Source: CAD feature listing. Evaluate the final solid. Frame: model axes, mm. A direction names the side the tool comes from. Give positions to 0.01 mm unless a question says otherwise; leave off trailing zeros. Write each loop counter-clockwise with the first axis right and the second up, starting at its lowest first coordinate (ties: lowest second). Pieces come first, ordered by that corner, then holes. Notation, with made-up numbers: (82, -3.5) - (100, -3.5) arc R21 cw to (100, 33.5) - close; hole circle Ø6 at (-31, 3). An arc over 180 degrees is marked (long way). One line per question, with ' | ' between items. Start each with the question number.
(1) Access query for faces 1 (the cylindrical face through (57.93, -6.22, 30.28)), 2 (the flat face through (47.3, -5, -13)), 3 (the flat face through (50, 11, -42)), 4 (the cylindrical face through (52.69, 14.39, 16.53)), 5 (the flat face through (-2, -5, 10)). Directions: +Z, -Z, +X, -X, +Y, -Y. A direction counts if a zero-diameter tool reaches every point of the face in a straight line with its end or side. Return the directions, or none.
(2) Pin query (flat end, axial travel): pin 1 (4 mm diameter, centred on x = -55, z = 45, fed in from +Y); pin 2 (3 mm diameter, centred on x = -55, z = -45, fed in from -Y); pin 3 (3 mm diameter, centred on x = 35, y = -0.5, fed in from +Z). Return the tip coordinate at first contact, or that it passes through.
(3) Draft query along Z for faces 6 (the conical face through (-54.6, 5.76, -43.12)), 7 (the flat face through (-60, 6, 1)), 8 (the flat face through (1, -1, -50)). Return one class per face: +Z half, -Z half, draft (parallel to the pull), parting line (faces both ways), or undercut.
(4) Section A-A, the plane z = 23.5. Return loops of the section in (x, y) (3 decimals), plus the area to 3 significant figures.
(5) Ray query, line 1 (Z direction, x = 55, y = 16); line 2 (Z direction, x = -55, y = 16.75); line 3 (X direction, y = 4, z = 42.5). Return the intervals inside material, ascending. Write a range as [from, to].
(6) Section D-D, the plane y = 10. State how many separate pieces and enclosed holes the cut face has, plus the area to 3 significant figures.
(7) Section B-B, the plane y = 3.5. Return loops of the section in (x, z).
(8) Section C-C, the plane x = -27.5. Return loops of the section in (y, z).
```python
from build123d import *

# Parameters (mm, degrees)
BOSS_EXTRUDE3_DEPTH       = 50
SKETCH7_W                 = 100
SKETCH7_H                 = 40
CUT_EXTRUDE1_DEPTH        = 11
SKETCH8_R                 = 3.96875
CUT_EXTRUDE2_DEPTH        = 121
CUT_EXTRUDE3_REACH        = 122
SKETCH9_W                 = 20
SKETCH9_H                 = 22
SKETCH10_R                = 3.175
CUT_EXTRUDE4_DEPTH        = 80
SKETCH11_W                = 12.7
SKETCH11_H                = 10
CUT_EXTRUDE5_DEPTH        = 15
F_5_0MM_DOWEL_HOLE1_D     = 5
F_5_0MM_DOWEL_HOLE1_DEPTH = 25
F_5_0MM_DOWEL_HOLE1_TIP   = 1.502151548
SKETCH15_R                = 2.5
CUT_EXTRUDE6_DEPTH        = 15


with BuildPart() as part:
    # Sketch6 → Boss-Extrude3 (new body, symmetric)
    with BuildSketch(Plane.XY):
        Polygon((-60, 22), (-50, 22), (-50, 0), (50, 0), (50, 22), (60, 22), (60, -10), (-60, -10), align=None)
    extrude(amount=BOSS_EXTRUDE3_DEPTH, both=True)

    # Sketch7 → Cut-Extrude1 (cut, through all)
    with BuildSketch(Plane(origin=(0, 0, 0), x_dir=(1, 0, 0), z_dir=(0, 1, 0))):
        with Locations((0, -30)):
            Rectangle(SKETCH7_W, SKETCH7_H)
    extrude(amount=-CUT_EXTRUDE1_DEPTH, mode=Mode.SUBTRACT)

    # Sketch8 → Cut-Extrude2 (cut, through all)
    with BuildSketch(Plane(origin=(60, 0, 0), x_dir=(0, 0, -1), z_dir=(1, 0, 0))):
        with Locations((-30, 10)):
            Circle(SKETCH8_R)
    extrude(amount=-CUT_EXTRUDE2_DEPTH, mode=Mode.SUBTRACT)

    # Sketch9 → Cut-Extrude3 (cut, up to next)
    with BuildSketch(Plane(origin=(60, 0, 0), x_dir=(0, 0, -1), z_dir=(1, 0, 0)), mode=Mode.PRIVATE) as cut_extrude3_sk1:
        with Locations((25, 11)):
            Rectangle(SKETCH9_W, SKETCH9_H)
    cut_extrude3_tool1 = extrude(cut_extrude3_sk1.sketch, amount=-CUT_EXTRUDE3_REACH, mode=Mode.PRIVATE) & part.part
    add(cut_extrude3_tool1.solids().sort_by_distance((60, 11, -25))[0], mode=Mode.SUBTRACT)

    # Sketch10 → Cut-Extrude4 (cut)
    with BuildSketch(Plane.XY.offset(50)):
        with Locations((55, -5)):
            Circle(SKETCH10_R)
    extrude(amount=-CUT_EXTRUDE4_DEPTH, mode=Mode.SUBTRACT)

    # Sketch11 → Cut-Extrude5 (cut)
    with BuildSketch(Plane.XZ.offset(10)):
        with Locations((53.65, 5)):
            Rectangle(SKETCH11_W, SKETCH11_H)
        with Locations((53.65, -12.5)):
            Rectangle(SKETCH11_W, SKETCH11_H)
    extrude(amount=-CUT_EXTRUDE5_DEPTH, mode=Mode.SUBTRACT)

    # Ø5.0mm Dowel Hole1
    with Locations(Plane(origin=(-676.293536786, 32, -1303.282701689), x_dir=(1, 0, 0), z_dir=(0, 1, 0))):
        with Locations((731.293536786, -1318.853535022), (621.293536786, -1318.853535022), (621.293536786, -1348.282701689), (621.293536786, -1259.995201689), (731.293536786, -1259.995201689), (731.293536786, -1296.570201689), (621.293536786, -1289.424368355)):
            Hole(F_5_0MM_DOWEL_HOLE1_D / 2, depth=F_5_0MM_DOWEL_HOLE1_DEPTH)
            with Locations((0, 0, -(F_5_0MM_DOWEL_HOLE1_DEPTH + F_5_0MM_DOWEL_HOLE1_TIP / 2))):  # 118° drill point
                Cone(0, F_5_0MM_DOWEL_HOLE1_D / 2, F_5_0MM_DOWEL_HOLE1_TIP, mode=Mode.SUBTRACT)

    # Sketch15 → Cut-Extrude6 (cut)
    with BuildSketch(Plane.XZ.offset(10)):
        with Locations((-55, -45)):
            Circle(SKETCH15_R)
        with Locations((-27.5, -45)):
            Circle(SKETCH15_R)
        with Locations((0, -45)):
            Circle(SKETCH15_R)
        with Locations((27.5, -45)):
            Circle(SKETCH15_R)
        with Locations((55, -45)):
            Circle(SKETCH15_R)
    extrude(amount=-CUT_EXTRUDE6_DEPTH, mode=Mode.SUBTRACT)


solid = part.part
```
Check sheet entries:
1) face 1: +Z | face 2: +X, +Y, -Y | face 3: +Z, -Z, +Y | face 4: +Y | face 5: +Z, +Y, -Y
2) pin 1: y = 6.7 | pin 2: y = 5 | pin 3: z = 10
3) face 6: undercut | face 7: draft | face 8: -Z half
4) outline: (-60, -10) - (-50, -10) - (-50, 22) - (-60, 22) - close; (50, -10) - (60, -10) - (60, 22) - (50, 22) - close; hole circle Ø6.35 at (55, -5) | area: 608 mm²
5) line 1: [-50, -45.79], [-40.79, -35], [-15, -9.21], [-4.21, 13.07], [18.07, 50] | line 2: [-50, -45.79], [-40.79, -16.36], [-11.36, 13.07], [18.07, 42.5], [47.5, 50] | line 3: [-60, -50], [50, 60]
6) separate pieces: 5 | enclosed holes: 7 | area: 1,500 mm²
7) outline: (-60, -50) - (-50, -50) - (-50, 50) - (-60, 50) - close; (50, -50) - (60, -50) - (60, -35) - (50, -35) - close; (50, -7.5) - (60, -7.5) - (60, 0) - (50, 0) - close; (50, 10) - (60, 10) - (60, 50) - (50, 50) - close; hole circle Ø5 at (-55, -45); hole circle Ø5 at (55, -45)
8) outline: (-10, -50) - (0, -50) - (0, -47.5) - (-10, -47.5) - close; (-10, -42.5) - (0, -42.5) - (0, 10) - (-10, 10) - close
